Part model, mm, in its own coordinate system. A direction names the side the tool comes from. Coordinates: 2 decimals unless noted, no trailing zeros. Loops run counter-clockwise (first coordinate to the right, second up) from the corner with the lowest first, then second, coordinate; pieces in that order, holes last. Notation, with made-up numbers: (82.5, 9.25) -> (132.5, 9.25) arc R11 ccw to (132.5, 17.25) -> close; hole circle Ø9 at (-27.5, 50). An arc over 180 degrees is marked (long way). One line per question, with ' | ' between items. Start each with the question number.
1) 3-axis set-ups, long thin cutter, end or side, ignore diameter. For faces 5 (the face through (32, 10.25, 2)), 6 (the face through (-35.035, 15, -1)), 7 (the face through (0, -7, -10)), 8 (the face through (41.978, 0.133, 3.915)), 9 (the face through (-12.248, 8.287, -5.07)): which of +Z, -Z, +X, -X, +Y, -Y reach the whole face in a straight line?
2) Drop flat-ended pins along their axis: pin 1 (0.9 mm diameter, centred on y = 14.5, z = -2, fed in from -X) (3 decimals); pin 2 (5 mm diameter, centred on x = -39.5, z = 2.5, fed in from -Y); pin 3 (5.5 mm diameter, centred on x = 31.82, y = 31.82, fed in from +Z); pin 4 (8 mm diameter, centred on x = 38, y = -38.5, fed in from +Z). Give the stop position or say it passes through.
3) Cut at B-B (z = -4.5). List the corners of the cut face in (x, y).
4) Cut at A-A (x = 0). List the corners of the cut face in (y, z) (3 decimals), plus the area to 3 significant figures.
5) Probe L1, parallel to Y at x = -10.5, z = -5.75; L2, parallel to Y at x = -10.5, z = 4.5 (3 decimals); L3, parallel to X at y = 1, z = -9. List the from-to ranges inside material, lowest first. Write a range as from..to.
6) Cut at C-C (x = 45). List the corners of the cut face in (y, z) (1 decimal).
7) Two-plate mould, pull along Y, no slides. Class faces 1 (the face through (-12, -23, -5)), 2 (the face through (12.287, 8.248, -5.07)), 3 (the face through (13, -7, -5)), 4 (the face through (-9, 0, 3.55)): released by +Y, released by -Y, zero draft, split by the parting line, or undercut.
8) Cut at D-D (y = 14.5). List the corners of the cut face in (x, z) (3 decimals).
from build123d import *

# Parameters (mm, degrees)
SKETCH_1_R                   = 50
EXTRUDE_1_DEPTH              = 5
SKETCH_13_W                  = 26
SKETCH_13_H                  = 32.5
EXTRUDE_3_DEPTH              = 10
FILLET_2_R                   = 2.5
SKETCH_6_R                   = 6.5
CUT_EXTRUDE_1_DEPTH          = 73.284161474
HOLE_WIZARD_M2_1_D           = 2.4
HOLE_WIZARD_M2_1_CBORE_D     = 3.85
HOLE_WIZARD_M2_1_CBORE_DEPTH = 1.45
HOLE_WIZARD_M3_2_D           = 3.4
HOLE_WIZARD_M3_2_CBORE_D     = 6.05
HOLE_WIZARD_M3_2_CBORE_DEPTH = 2.2
PATTERN_CIRCULAR_1_COUNT     = 8
SKETCH_7_W                   = 3
SKETCH_7_H                   = 3
EXTRUDE_2_DEPTH              = 3
FILLET_1_R                   = 1
FILLET_1_OF_MIRROR_2_R       = 1
SKETCH_9_W                   = 5
SKETCH_9_H                   = 2
CUT_EXTRUDE_2_DEPTH          = 72.414284285
HOLE_WIZARD_M3_3_D           = 3.4
HOLE_WIZARD_M3_3_CBORE_D     = 6.05
HOLE_WIZARD_M3_3_CBORE_DEPTH = 2.2


with BuildPart() as part:
    # ｽｹｯﾁ1 → ﾎﾞｽ - 押し出し1 (new body)
    with BuildSketch(Plane.XY):
        Circle(SKETCH_1_R)
    extrude(amount=EXTRUDE_1_DEPTH)

    # ｽｹｯﾁ13 → ﾎﾞｽ - 押し出し3 (add)
    with BuildSketch(Plane(origin=(0, 0, 0), x_dir=(-1, 0, 0), z_dir=(0, 0, -1))):
        with Locations((0, -7.25)):
            Rectangle(SKETCH_13_W, SKETCH_13_H)
    extrude(amount=EXTRUDE_3_DEPTH)

    # ﾌｨﾚｯﾄ2
    fillet_2_edges = [part.edges().sort_by_distance(p)[0] for p in [
        (13, 9, -5),
        (13, -23.5, -5),
        (-13, -23.5, -5),
        (-13, 9, -5),
    ]]
    fillet(fillet_2_edges, radius=FILLET_2_R)

    # ｽｹｯﾁ6 → ｶｯﾄ - 押し出し1 (cut, through all)
    with BuildSketch(Plane.XY.offset(5)):
        Circle(SKETCH_6_R)
    extrude(amount=-CUT_EXTRUDE_1_DEPTH, mode=Mode.SUBTRACT)

    # M2 丸平ねじ用座ぐり穴1 (through all)
    with Locations(Plane.XY.offset(5)):
        with Locations((-10.5, 0), (-10.5, -21)):
            hole_wizard_m2_1 = CounterBoreHole(HOLE_WIZARD_M2_1_D / 2, HOLE_WIZARD_M2_1_CBORE_D / 2, HOLE_WIZARD_M2_1_CBORE_DEPTH)

    # ﾐﾗｰ1: M2 丸平ねじ用座ぐり穴1 across plane
    add(hole_wizard_m2_1.mirror(Plane(origin=(0, 0, 0), x_dir=(0, 0, 1), z_dir=(1, 0, 0))), mode=Mode.SUBTRACT)

    # M3 丸平ねじ用座ぐり穴2 (through all)
    with Locations(Plane.XY.offset(5)):
        with Locations((45, 0)):
            hole_wizard_m3_2 = CounterBoreHole(HOLE_WIZARD_M3_2_D / 2, HOLE_WIZARD_M3_2_CBORE_D / 2, HOLE_WIZARD_M3_2_CBORE_DEPTH)

    # 円形ﾊﾟﾀｰﾝ1: M3 丸平ねじ用座ぐり穴2 ×8 about axis
    pattern_circular_1_axis = Axis((0, 0, 0), (0, 0, 1))
    for i in range(1, PATTERN_CIRCULAR_1_COUNT):
        add(hole_wizard_m3_2.rotate(pattern_circular_1_axis, i * 360 / PATTERN_CIRCULAR_1_COUNT), mode=Mode.SUBTRACT)

    # ｽｹｯﾁ7 → ﾎﾞｽ - 押し出し2 (add)
    with BuildSketch(Plane(origin=(0, 0, 0), x_dir=(-1, 0, 0), z_dir=(0, 0, -1))):
        with Locations((36.535, 14.75)):
            Rectangle(SKETCH_7_W, SKETCH_7_H)
    extrude_2 = extrude(amount=EXTRUDE_2_DEPTH)

    # ﾌｨﾚｯﾄ1
    fillet_1_edges = [part.edges().sort_by_distance(p)[0] for p in [
        (-38.035, 14.75, 0),
    ]]
    fillet(fillet_1_edges, radius=FILLET_1_R)

    # ﾐﾗｰ2: ﾎﾞｽ - 押し出し2 across plane
    add(extrude_2.mirror(Plane(origin=(0, 0, 0), x_dir=(0, 0, 1), z_dir=(1, 0, 0))))

    # ﾌｨﾚｯﾄ1 of ﾐﾗｰ2
    fillet_1_of_mirror_2_edges = [part.edges().sort_by_distance(p)[0] for p in [
        (38.035, 14.75, 0),
    ]]
    fillet(fillet_1_of_mirror_2_edges, radius=FILLET_1_OF_MIRROR_2_R)

    # ｽｹｯﾁ9 → ｶｯﾄ - 押し出し2 (cut, through all)
    with BuildSketch(Plane(origin=(0, 0, 0), x_dir=(-1, 0, 0), z_dir=(0, 0, -1))):
        with Locations((31.535, 16.85)):
            Rectangle(SKETCH_9_W, SKETCH_9_H)
        with Locations((31.535, 11.25)):
            Rectangle(SKETCH_9_W, SKETCH_9_H)
    cut_extrude_2 = extrude(amount=-CUT_EXTRUDE_2_DEPTH, mode=Mode.SUBTRACT)

    # ﾐﾗｰ3: ｶｯﾄ - 押し出し2 across plane
    add(cut_extrude_2.mirror(Plane(origin=(0, 0, 0), x_dir=(0, 0, 1), z_dir=(1, 0, 0))), mode=Mode.SUBTRACT)

    # M3 丸平ねじ用座ぐり穴3 (through all)
    with Locations(Plane.XY.offset(5)):
        with Locations((-20, -5)):
            CounterBoreHole(HOLE_WIZARD_M3_3_D / 2, HOLE_WIZARD_M3_3_CBORE_D / 2, HOLE_WIZARD_M3_3_CBORE_DEPTH)


solid = part.part
Reported:
1) face 5: +Z, -Z | face 6: -Z, +Y, -Y | face 7: -Z, +X, -X, +Y, -Y | face 8: +Z | face 9: -Z, -X, +Y
2) pin 1: stops at x = -38.035 | pin 2: stops at y = -33.63 | pin 3: stops at z = 2.8 | pin 4: passes through
3) outline: (-13, -21) arc R2.5 ccw to (-10.5, -23.5) -> (10.5, -23.5) arc R2.5 ccw to (13, -21) -> (13, 6.5) arc R2.5 ccw to (10.5, 9) -> (-10.5, 9) arc R2.5 ccw to (-13, 6.5) -> close; hole circle Ø2.4 at (-10.5, -21); hole circle Ø2.4 at (-10.5, 0); hole circle Ø13 at (0, 0); hole circle Ø2.4 at (10.5, -21); hole circle Ø2.4 at (10.5, 0)
4) outline: (-50, 0) -> (-46.7, 0) -> (-46.7, 2.8) -> (-48.025, 2.8) -> (-48.025, 5) -> (-50, 5) -> close; (-43.3, 0) -> (-23.5, 0) -> (-23.5, -10) -> (-6.5, -10) -> (-6.5, 5) -> (-41.975, 5) -> (-41.975, 2.8) -> (-43.3, 2.8) -> close; (6.5, -10) -> (9, -10) -> (9, 0) -> (43.3, 0) -> (43.3, 2.8) -> (41.975, 2.8) -> (41.975, 5) -> (6.5, 5) -> close; (46.7, 0) -> (50, 0) -> (50, 5) -> (48.025, 5) -> (48.025, 2.8) -> (46.7, 2.8) -> close | area: 584 mm²
5) L1: y = -23.5..-22.2, -19.8..-1.2, 1.2..9 | L2: y = -48.885..-22.925, -19.075..-1.925, 1.925..48.885 | L3: x = -13..-11.16, -9.84..-6.42, 6.42..9.84, 11.16..13
6) outline: (-21.8, 0) -> (-1.7, 0) -> (-1.7, 2.8) -> (-3, 2.8) -> (-3, 5) -> (-21.8, 5) -> close; (1.7, 0) -> (21.8, 0) -> (21.8, 5) -> (3, 5) -> (3, 2.8) -> (1.7, 2.8) -> close
7) face 1: released by -Y | face 2: released by +Y | face 3: zero draft | face 4: undercut
8) outline: (-47.851, 0) -> (-39.035, 0) arc R1 cw to (-38.035, -1) -> (-38.035, -3) -> (-35.035, -3) -> (-35.035, 0) -> (35.035, 0) -> (35.035, -3) -> (38.035, -3) -> (38.035, -1) arc R1 cw to (39.035, 0) -> (47.851, 0) -> (47.851, 5) -> (-47.851, 5) -> close
